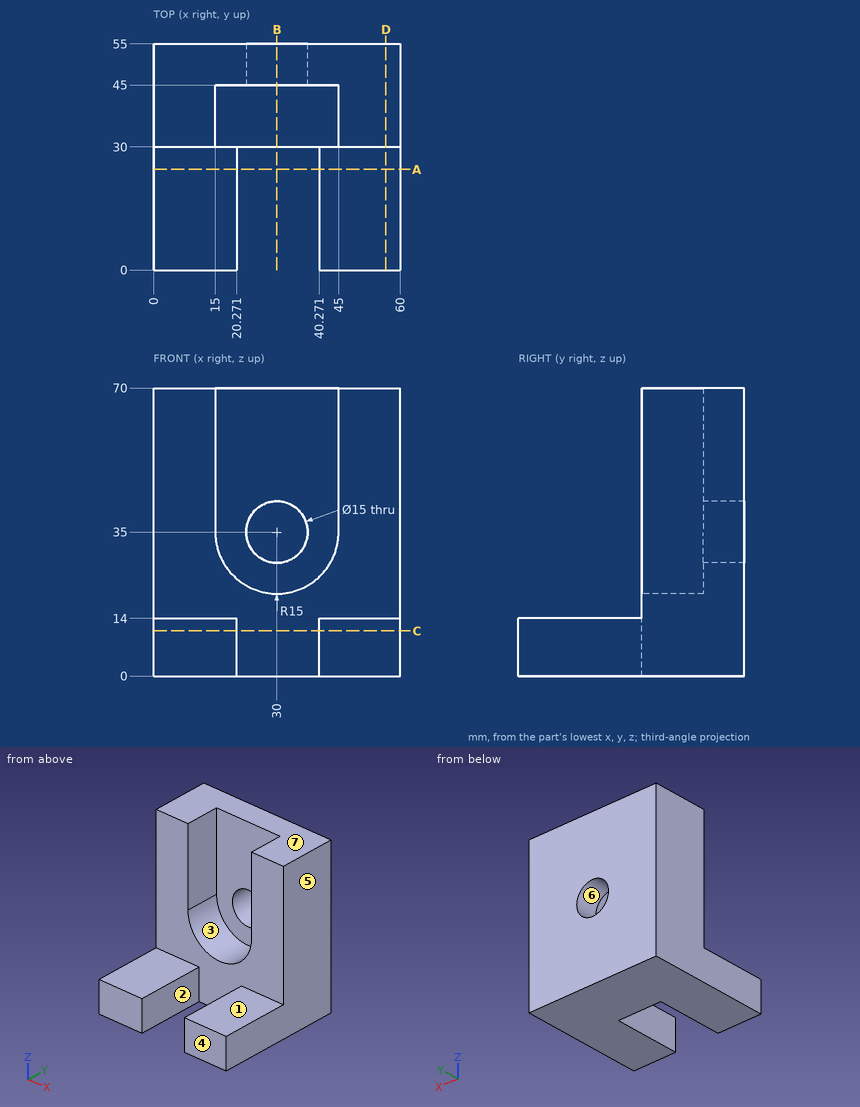
Check sheet for the drawn part. Datum: minimum x, y, z corner. Units: mm. A direction names the side the tool comes from. Coordinates: 2 decimals unless noted, no trailing zeros. Write each loop counter-clockwise with the first axis right and the second up, starting at its lowest first coordinate (ties: lowest second). Pieces come first, ordered by that corner, then holes. Notation, with made-up numbers: M -19,26 L 18,26 A21 cw 18,65 Z; hole C 82,80.5 d7. An arc over 180 degrees is marked long. Use a Markdown table: item, result.
Q1. Sectioned sample at B-B, the plane x = 30. Record the boundary of the cut face in (y, z).
Reply:
| item | result |
|---|---|
| outline | M 30,0 L 55,0 L 55,27.5 L 45,27.5 L 45,20 L 30,20 Z; M 45,42.5 L 55,42.5 L 55,70 L 45,70 Z |
Q2. Go/stop test with flat-tipped pins: P1, Ø9, axis at x = 29, z = 51.5, coming from the -Y side; P2, Ø12, axis at x = 37, y = 27, coming from the +Z side; P3, Ø22.5, axis at x = 11.5, y = 18, coming from the +Z side; P4, Ø9, axis at x = 30, z = 35, coming from the +Y side. Record where each tip stops, or that it passes through.
Reply:
| item | result |
|---|---|
| P1 | stops at y = 45 |
| P2 | stops at z = 26.27 |
| P3 | stops at z = 14 |
| P4 | passes through |
Q3. Draft check along Z on the marked faces 5, 6 and 7. Enter one of: +Z half, -Z half, draft (parallel to the pull), parting line (faces both ways), or undercut.
Reply:
| item | result |
|---|---|
| face 5 | draft |
| face 6 | undercut |
| face 7 | +Z half |
Q4. Thickness scan on line 1 (X direction, y = 50.5, z = 35); line 2 (X direction, y = 35, z = 66); line 3 (Z direction, x = 30, y = 48). Record the ranges inside material, lowest first.
Reply:
| item | result |
|---|---|
| line 1 | x = 0 to 22.5, 37.5 to 60 |
| line 2 | x = 0 to 15, 45 to 60 |
| line 3 | z = 0 to 27.5, 42.5 to 70 |
Q5. Set-up check for the marked faces 1, 2, 3 and 4: record each of +Z, -Z, +X, -X, +Y, -Y from which the full face is reachable in a straight line by a thin tool's end or side.
Reply:
| item | result |
|---|---|
| face 1 | +Z, +X, -X, -Y |
| face 2 | +Z, -Z, -Y |
| face 3 | +Z, -Y |
| face 4 | +Z, -Z, +X, -X, -Y |
Q6. Sectioned sample at D-D, the plane x = 56.5. Record the boundary of the cut face in (y, z), plus the area to 3 significant figures.
Reply:
| item | result |
|---|---|
| outline | M 0,0 L 55,0 L 55,70 L 30,70 L 30,14 L 0,14 Z |
| area | 2,170 mm² |
Q7. Sectioned sample at C-C, the plane z = 11. Record the boundary of the cut face in (x, y).
Reply:
| item | result |
|---|---|
| outline | M 0,0 L 20.27,0 L 20.27,30 L 40.27,30 L 40.27,0 L 60,0 L 60,55 L 0,55 Z |
Q8. Sectioned sample at A-A, the plane y = 24.5. Record the boundary of the cut face in (x, z), plus the area to 3 significant figures.
Reply:
| item | result |
|---|---|
| outline | M 0,0 L 20.27,0 L 20.27,14 L 0,14 Z; M 40.27,0 L 60,0 L 60,14 L 40.27,14 Z |
| area | 560 mm² |
